Geometry check sheet. Reference: the model listing, model coordinates, mm. Face numbers are marked on the shaded views. A direction names the side the tool comes from. Give positions to 0.01 mm unless a question says otherwise; leave off trailing zeros. Loops run counter-clockwise (first coordinate to the right, second up) from the corner with the lowest first, then second, coordinate; pieces in that order, holes last.
1. Material ranges on L1, parallel to X at y = 1.75, z = 7.75; L2, parallel to Y at x = -0.5, z = 0.75; L3, parallel to Y at x = 0.75, z = 2.5, recorded low to high.
2. Cross-section at A-A, the plane x = -0.25. Record the cut outline in (y, z), plus the area to 3 significant figures.
3. Cross-section at B-B, the plane z = 0.75. Record the cut outline in (x, y).
4. Cross-section at D-D, the plane z = 7. Record the cut outline in (x, y), plus the area to 3 significant figures.
5. Cross-section at C-C, the plane x = 1.25. Record the cut outline in (y, z).
6. Tool access check on the marked faces 4 and 5. Record the directions out of +Z, -Z, +X, -X, +Y, -Y that give a thin tool (end or side, any length) a straight path to the whole face; none if there is none.
7. Release check for a two-part mould opening along Y. For the marked faces 1, 2 and 3 record: +Y half, -Y half, draft (parallel to the pull), parting line (faces both ways), or undercut.
8. Go/stop test with flat-tipped pins: pin 1 Ø0.6 at (x, z) = (0, 2.5) entering from -Y; pin 2 Ø1.5 at (x, z) = (4.5, 6.5) entering from +Y. Record where each tip stops, or that it passes through.
from build123d import *

# Parameters (mm, degrees)
SKETCH1_W      = 12
SKETCH1_H      = 17
SKETCH1_W_2    = 2
SKETCH1_H_2    = 4.2
EXTRUDE1_DEPTH = 8
EXTRUDE2_DEPTH = 17.740669043
FILLET1_R      = 10


with BuildPart() as part:
    # Sketch1 → Extrude1 (new body)
    with BuildSketch(Plane.XY):
        Rectangle(SKETCH1_W, SKETCH1_H)
        Rectangle(SKETCH1_W_2, SKETCH1_H_2, mode=Mode.SUBTRACT)
    extrude(amount=EXTRUDE1_DEPTH)

    # Sketch2 → Extrude2 (cut, through all)
    with BuildSketch(Plane.ZY.offset(6)):
        Polygon((2, 8.5), (3.349347136, 4.792699212), (8, 3.1), (8, 8.5), align=None)
    extrude2 = extrude(amount=-EXTRUDE2_DEPTH, mode=Mode.SUBTRACT)

    # Mirror1: Extrude2 across plane
    add(extrude2.mirror(Plane.ZX), mode=Mode.SUBTRACT)

    # Fillet1
    # the kernel refuses this fillet: 10 mm, written as the material it adds along each edge
    with BuildSketch(Plane(origin=(-6, -4.792699212, 3.349347136), x_dir=(0, -0.9396926207859071, -0.34202014332567254), z_dir=(1, 0, 0))) as fillet1_piece_1:
        with BuildLine():
            CenterArc((4.686139514, -9.972514667), FILLET1_R, 94.249009028, 45.750990972)
            Line((-2.974304917, -3.54463857), (-3.127513806, -3.416081048))
            Line((-3.127513806, -3.416081048), (-0.153208889, 0.128557522))
            Line((-0.153208889, 0.128557522), (0, 0.2))
            ThreePointArc((0, 0.2), (1.972613547, 0.2), (3.930408846, 0.199450293))
            Line((3.930408846, 0.199450293), (3.945227094, 0))
        make_face()
    extrude(amount=12)
    with BuildSketch(Plane(origin=(-6, 4.792699212, 3.349347136), x_dir=(0, 0.9396926207859071, -0.34202014332567254), z_dir=(1, 0, 0))) as fillet1_piece_2:
        with BuildLine():
            CenterArc((4.686139514, 9.972514667), FILLET1_R, 220, 45.750990972)
            Line((-2.974304917, 3.54463857), (-3.127513806, 3.416081048))
            Line((-3.127513806, 3.416081048), (-0.153208889, -0.128557522))
            Line((-0.153208889, -0.128557522), (0, -0.2))
            ThreePointArc((0, -0.2), (1.972613547, -0.2), (3.930408846, -0.199450293))
            Line((3.930408846, -0.199450293), (3.945227094, 0))
        make_face()
    extrude(amount=12)


solid = part.part
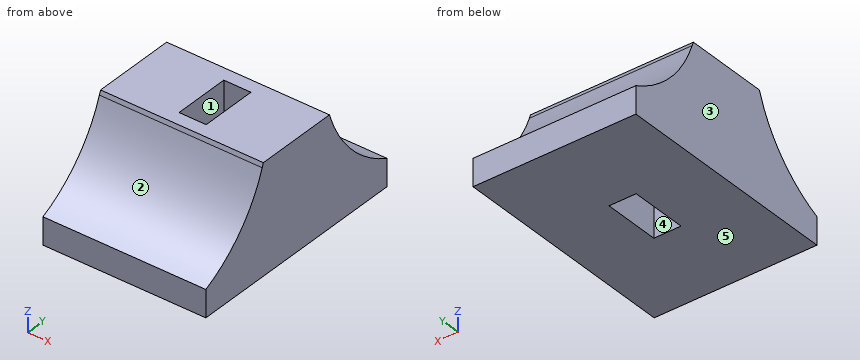
Result:
1. L1: x = -6 to -1, 1 to 6
1. L2: y = -8.5 to -2.1, 2.1 to 8.5
1. L3: y = -7.53 to -2.1, 2.1 to 7.53
2. outline: (-8.5, 0) - (-2.1, 0) - (-2.1, 8) - (-3.1, 8) - (-3.21, 7.7) arc R10 cw to (-8.5, 2) - close; (2.1, 0) - (8.5, 0) - (8.5, 2) arc R10 cw to (3.21, 7.7) - (3.1, 8) - (2.1, 8) - close
2. area: 60.8 mm2
3. outline: (-6, -8.5) - (6, -8.5) - (6, 8.5) - (-6, 8.5) - close; hole (-1, -2.1) - (1, -2.1) - (1, 2.1) - (-1, 2.1) - close
4. outline: (-6, -3.49) - (6, -3.49) - (6, 3.49) - (-6, 3.49) - close; hole (-1, -2.1) - (1, -2.1) - (1, 2.1) - (-1, 2.1) - close
4. area: 75.5 mm2
5. outline: (-8.5, 0) - (8.5, 0) - (8.5, 2) arc R10 cw to (3.21, 7.7) - (3.1, 8) - (-3.1, 8) - (-3.21, 7.7) arc R10 cw to (-8.5, 2) - close
6. face 4: +Z, -Z
6. face 5: -Z, +X, -X, +Y, -Y
7. face 1: undercut
7. face 2: -Y half
7. face 3: draft
8. pin 1: stops at y = -8.08
8. pin 2: stops at y = 4.17
